Autodesk Inventor part; units mm, degrees
ref_plane "YZ Plane" through (0, 0, 0) normal (1, 0, 0) x (0, 1, 0)
ref_plane "XZ Plane" through (0, 0, 0) normal (0, 1, 0) x (-1, 0, 0)
ref_plane "XY Plane" through (0, 0, 0) normal (0, 0, 1) x (1, 0, 0)
sketch "Sketch1" plane through (0, 0, 0) normal (0, 1, 0) x (-1, 0, 0)
  circle A0 centre (0, 0) radius 7
  circle A1 centre (0, 0) radius 8
  dimension "d0" = 14
  dimension "d1" = 1
extrude "Extrusion1" add sketch "Sketch1" along normal blind 10.5
sketch "Sketch2" plane through (0, 0, 0) normal (0, -1, 0) x (1, 0, 0)
  circle A0 centre (0, 0) radius 8
extrude "Extrusion2" [suppressed]
sketch "Sketch4" plane through (0, 10.5, 0) normal (0, 1, 0) x (1, 0, 0)
  circle A0 centre (-10, 0) radius 1.25
  circle A1 centre (-10, 0) radius 2.5
  point P0 (0, 0)
  dimension "d6" = 5
  dimension "d7" = 2.5
  dimension "d8" = 10
extrude "Extrusion3" add sketch "Sketch4" against normal up to surface (10.5 mm away)
pattern_circular "Circular Pattern1" count 4 over 360 about axis through (0, 0, 0) along (0, 1, 0) of "Extrusion3"
fillet "Fillet1" radius 1 8 edges at (7.8875, 5.25, -1.3369) (7.8875, 5.25, 1.3369) (1.3369, 5.25, 7.8875) (-1.3369, 5.25, 7.8875) (-7.8875, 5.25, 1.3369) (-7.8875, 5.25, -1.3369) (-1.3369, 5.25, -7.8875) (1.3369, 5.25, -7.8875)
sketch "Sketch5" plane through (0, 0, 0) normal (0, -1, 0) x (1, 0, 0)
  line L0 (-15, -15) -> (15, -15)
  line L1 (15, -15) -> (15, 15)
  line L2 (15, 15) -> (-15, 15)
  line L3 (-15, 15) -> (-15, -15)
  line L4 (-15, -15) -> (15, 15) construction
  line L5 (15, -15) -> (-15, 15) construction
  point P0 (0, 0)
  dimension "d23" = 30
  dimension "d24" = 30
extrude "Extrusion4" add sketch "Sketch5" along normal blind 4
sketch "Sketch6" plane through (0, -4, 0) normal (0, 1, 0) x (1, 0, 0)
  line L0 (15, 15) -> (15, -15)
  line L1 (-15, -15) -> (15, -15)
  line L2 (15, -15) -> (15, 15)
  line L3 (15, 15) -> (-15, 15)
  line L4 (-15, 15) -> (-15, -15)
  line L5 (-15, -15) -> (15, 15) construction
  line L6 (15, -15) -> (-15, 15) construction
  line L7 (-19, -19) -> (19, -19)
  line L8 (19, -19) -> (19, 19)
  line L9 (19, 19) -> (-19, 19)
  line L10 (-19, 19) -> (-19, -19)
  line L11 (-19, -19) -> (19, 19) construction
  line L12 (19, -19) -> (-19, 19) construction
  point P0 (0, 0)
  dimension "d27" = 4
  dimension "d28" = 4
extrude "Extrusion5" add sketch "Sketch6" along normal blind 18.5
fillet "Fillet2" radius 2 8 edges at (-15, 7.25, -15) (15, 7.25, -15) (-15, 7.25, 15) (15, 7.25, 15) (19, 5.25, 19) (19, 5.25, -19) (-19, 5.25, 19) (-19, 5.25, -19)
properties part number "Ecoflex_mould"
Build history of the part. All positions in model axes, mm. A direction names the side the tool comes from. Round coordinates to 2 decimals unless told otherwise and drop trailing zeros. Write each loop counter-clockwise with the first axis right and the second up, starting at its lowest first coordinate (ties: lowest second). Pieces come first, ordered by that corner, then holes. Notation, with made-up numbers: (76, 26) - (117, 26) arc R28 cw to (117, 62) - close; hole circle Ø5 at (51, 2.25). An arc over 180 degrees is marked (long way). One line per question, with ' | ' between items.
1. Band-saw the part on A-A, the plane y = 12.5. Write the cut outline in (x, z), and give its area (3 significant figures).
Results are:
outline: (-19, -17) arc R2 ccw to (-17, -19) - (17, -19) arc R2 ccw to (19, -17) - (19, 17) arc R2 ccw to (17, 19) - (-17, 19) arc R2 ccw to (-19, 17) - close; hole (-15, -13) arc R2 ccw to (-13, -15) - (13, -15) arc R2 ccw to (15, -13) - (15, 13) arc R2 ccw to (13, 15) - (-13, 15) arc R2 ccw to (-15, 13) - close | area: 544 mm^2
2. Mould opens along X. For faces 3 (the face through (18.43, 5.38, -18.4)), 4 (the face through (-12.5, 5.3, -0.1)), 5 (the face through (17, 14.5, 0)) say: released by +X, released by -X, zero draft, split by the parting line, or undercut.
Results are:
face 3: released by +X | face 4: undercut | face 5: zero draft
3. Drill centre lines: line 1 along Z through (x, y) = (10, 2.75); line 2 along Z through (x, y) = (7.5, 11.5). Where is each one in solid material? Low to high. Write a range as from..to.
Results are:
line 1: -19..-15, -2.5..-1.25, 1.25..2.5, 15..19 | line 2: -19..-15, 15..19
4. Drop flat-ended pins along their axis: pin 1 Ø3 at (x, z) = (10.5, 0) entering from +Y; pin 2 Ø12.5 at (x, z) = (0, 0) entering from +Y. Give the stop position or say it passes through.
Results are:
pin 1: y = 10.5 | pin 2: y = 0
5. Tool access for faces 1 (the face through (10, 0, 0)), 2 (the face through (-18.4, 5.38, -18.43)): list every direction of +Z, -Z, +X, -X, +Y, -Y with a clear straight run to the whole face (end or side of a thin tool).
Results are:
face 1: +Y | face 2: -Z, -X, +Y, -Y
6. Band-saw the part on C-C, the plane z = -10. Write the cut outline in (x, y), and give its area (3 significant figures).
Results are:
outline: (-19, -4) - (19, -4) - (19, 14.5) - (15, 14.5) - (15, 0) - (2.5, 0) - (2.5, 10.5) - (1.25, 10.5) - (1.25, 0) - (-1.25, 0) - (-1.25, 10.5) - (-2.5, 10.5) - (-2.5, 0) - (-15, 0) - (-15, 14.5) - (-19, 14.5) - close | area: 294 mm^2
7. Band-saw the part on D-D, the plane y = 4.5. Give the number of separate pieces and of enclosed holes in the cut face, and give its area (3 significant figures).
Results are:
separate pieces: 2 | enclosed holes: 6 | area: 650 mm^2
8. Band-saw the part on B-B, the plane x = 0. Write the cut outline in (y, z), and give its area (3 significant figures).
Results are:
outline: (-4, -19) - (14.5, -19) - (14.5, -15) - (0, -15) - (0, -12.5) - (10.5, -12.5) - (10.5, -11.25) - (0, -11.25) - (0, -8.75) - (10.5, -8.75) - (10.5, -7) - (0, -7) - (0, 7) - (10.5, 7) - (10.5, 8.75) - (0, 8.75) - (0, 11.25) - (10.5, 11.25) - (10.5, 12.5) - (0, 12.5) - (0, 15) - (14.5, 15) - (14.5, 19) - (-4, 19) - close | area: 331 mm^2
